```python
from build123d import *

# Parameters (mm, degrees)
SKETCH1_R           = 1.5
BOSS_EXTRUDE1_DEPTH = 2
SKETCH2_W           = 13
SKETCH2_H           = 10
BOSS_EXTRUDE2_DEPTH = 6
SKETCH3_R           = 2.5
BOSS_EXTRUDE3_DEPTH = 10
FILLET1_R           = 2.5


with BuildPart() as part:
    # Sketch1 → Boss-Extrude1 (new body)
    with BuildSketch(Plane(origin=(0, 0, 0), x_dir=(1, 0, 0), z_dir=(0, 1, 0))):
        with BuildLine():
            Line((-12, 11), (12, 11))
            ThreePointArc((12, 11), (14.121320344, 10.121320344), (15, 8))
            Line((15, 8), (15, -8))
            ThreePointArc((15, -8), (14.121320344, -10.121320344), (12, -11))
            Line((12, -11), (-12, -11))
            ThreePointArc((-12, -11), (-14.121320344, -10.121320344), (-15, -8))
            Line((-15, -8), (-15, 8))
            ThreePointArc((-15, 8), (-14.121320344, 10.121320344), (-12, 11))
        make_face()
        with Locations(Location((12, 8, 0), (0, 0, 270))):
            Circle(SKETCH1_R, mode=Mode.SUBTRACT)
        with Locations(Location((12, -8, 0), (0, 0, 270))):
            Circle(SKETCH1_R, mode=Mode.SUBTRACT)
    extrude(amount=BOSS_EXTRUDE1_DEPTH)

    # Sketch2 → Boss-Extrude2 (add)
    with BuildSketch(Plane(origin=(0, 2, 0), x_dir=(1, 0, 0), z_dir=(0, 1, 0))):
        with Locations((-15.5, 0)):
            Rectangle(SKETCH2_W, SKETCH2_H)
    extrude(amount=BOSS_EXTRUDE2_DEPTH)

    # Sketch3 → Boss-Extrude3 (add)
    with BuildSketch(Plane(origin=(0, 2, 0), x_dir=(1, 0, 0), z_dir=(0, 1, 0))):
        with Locations(Location((3, 0, 0), (0, 0, 270))):
            Circle(SKETCH3_R)
    extrude(amount=BOSS_EXTRUDE3_DEPTH)

    # Fillet1
    fillet1_edges = [part.edges().sort_by_distance(p)[0] for p in [
        (3, 12, -2.5),
    ]]
    fillet(fillet1_edges, radius=FILLET1_R)


solid = part.part
```
Geometry: final body of the model. Coordinates: model frame, mm. A direction names the side the tool comes from. Coordinates: 2 decimals unless noted, no trailing zeros. Order: outer loops, then holes, each group sorted by start corner. A loop starts at its lowest first (then second) coordinate and runs counter-clockwise, first axis right, second up. Notation, with made-up numbers: (63, 53.25) -> (75, 53.25) arc R18 cw to (75, 59.25) -> close; hole circle Ø6 at (-23.5, 55.25). An arc over 180 degrees is marked (long way). Answer in a Markdown table with one row per item.
Item 1: Draft query along X for faces 5 (the flat face through (-9, 5, 0)), 6 (the flat face through (-16, 5, -5)), 7 (the cylindrical face through (14.1, 0.99, -10.14)), 8 (the cylindrical face through (12.07, 0.99, -9.5)). Return one class per face: released by +X, released by -X, zero draft, split by the parting line, or undercut.
Return value:
| item | result |
|---|---|
| face 5 | undercut |
| face 6 | zero draft |
| face 7 | released by +X |
| face 8 | undercut |
Item 2: Section A-A on y = 4.25. Output: boundary loops of the cut face in (x, z).
Return value:
| item | result |
|---|---|
| outline | (-22, -5) -> (-9, -5) -> (-9, 5) -> (-22, 5) -> close; circle Ø5 at (3, 0) |
Item 3: Section C-C on x = 3. Output: boundary loops of the cut face in (y, z).
Return value:
| item | result |
|---|---|
| outline | (0, -11) -> (2, -11) -> (2, -2.5) -> (9.5, -2.5) arc R2.5 ccw to (9.5, 2.5) -> (2, 2.5) -> (2, 11) -> (0, 11) -> close |
Item 4: Section D-D on y = 8.75. Output: boundary loops of the cut face in (x, z).
Return value:
| item | result |
|---|---|
| outline | circle Ø5 at (3, 0) |
Item 5: Contact query for flat-ended pins moving along their axis: P1, Ø2, axis at x = -19, z = -1.5, coming from the -Y side; P2, Ø1.5, axis at x = 1, y = 4, coming from the -Z side; P3, Ø5, axis at x = 12, z = -8, coming from the +Y side; P4, Ø1, axis at x = 7.5, y = 5, coming from the -Z side. Output: stop coordinate, or through.
Return value:
| item | result |
|---|---|
| P1 | stops at y = 2 |
| P2 | stops at z = -2.17 |
| P3 | stops at y = 2 |
| P4 | passes through |
Item 6: Ray query, L1, parallel to X at y = 0.85, z = 8; L2, parallel to X at y = 0.75, z = 3; L3, parallel to Y at x = -2, z = 8. Return the intervals inside material, ascending.
Return value:
| item | result |
|---|---|
| L1 | x = -15 to 10.5, 13.5 to 15 |
| L2 | x = -15 to 15 |
| L3 | y = 0 to 2 |
Item 7: Access query for faces 1 (the cylindrical face through (0.56, 5.7, -0.54)), 2 (the flat face through (-16, 8, 0)), 3 (the flat face through (-16, 5, 5)), 4 (the flat face through (-19, 2, 0)). Directions: +Z, -Z, +X, -X, +Y, -Y. A direction counts if a zero-diameter tool reaches every point of the face in a straight line with its end or side. Return the directions, or none.
Return value:
| item | result |
|---|---|
| face 1 | +Y |
| face 2 | +Z, -Z, -X, +Y |
| face 3 | +Z, +X, -X, +Y |
| face 4 | +Z, -Z, -X, -Y |
Item 8: Section B-B on z = 0. Output: boundary loops of the cut face in (x, y), plus the area to 3 significant figures.
Return value:
| item | result |
|---|---|
| outline | (-22, 2) -> (-15, 2) -> (-15, 0) -> (15, 0) -> (15, 2) -> (5.5, 2) -> (5.5, 9.5) arc R2.5 ccw to (0.5, 9.5) -> (0.5, 2) -> (-9, 2) -> (-9, 8) -> (-22, 8) -> close |
| area | 185 mm² |
